```python
from build123d import *

# Parameters (mm, degrees)
MASS_DEPTH                = 6.35
SKETCH4_R                 = 9.271
CUT_EXTRUDE1_DEPTH        = 54.623672769
SKETCH3_W                 = 9.525
SKETCH3_H                 = 12.7
CUT_EXTRUDE2_DEPTH        = 54.623672769
LPATTERN1_COUNT           = 2
LPATTERN1_PITCH           = 19.05
CAVITY1_START             = -19.1516
CAVITY1_OUTLINE_W         = 11.1125
CAVITY1_OUTLINE_H         = 6.35
CAVITY1_DEPTH             = 6.35
CAVITY1_START_2           = 12.7
CAVITY1_2_OUTLINE_W       = 11.1125
CAVITY1_2_OUTLINE_H       = 6.35
CAVITY1_2_DEPTH           = 6.35
SKETCH5_R                 = 7.9375
CUT_EXTRUDE3_DEPTH        = 54.623672769
F_6_32_TAPPED_HOLE1_D     = 2.7051
F_6_32_TAPPED_HOLE1_DEPTH = 152.4
F_6_32_TAPPED_HOLE1_TIP   = 0.81269403


# Read off the part's stored shape, not the designer's step: Cavity1
with BuildPart() as part:
    # Sketch1 → Mass (new body)
    with BuildSketch(Plane.XY):
        with BuildLine():
            Line((-19.05, -23.8125), (19.05, -23.8125))
            Line((19.05, -23.8125), (19.05, 23.8125))
            Line((19.05, 23.8125), (-19.05, 23.8125))
            Line((-19.05, 23.8125), (-38.68314018, 14.281008096))
            ThreePointArc((-38.68314018, 14.281008096), (-47.625, 0), (-38.68314018, -14.281008096))
            Line((-38.68314018, -14.281008096), (-19.05, -23.8125))
        make_face()
    extrude(amount=MASS_DEPTH)

    # Sketch4 → Cut-Extrude1 (cut, through all)
    with BuildSketch(Plane(origin=(0, 0, 0), x_dir=(-1, 0, 0), z_dir=(0, 0, -1))):
        with Locations((31.75, 0)):
            Circle(SKETCH4_R)
    extrude(amount=-CUT_EXTRUDE1_DEPTH, mode=Mode.SUBTRACT)

    # Sketch3 → Cut-Extrude2 (cut, through all)
    with BuildSketch(Plane(origin=(0, 0, 0), x_dir=(-1, 0, 0), z_dir=(0, 0, -1))):
        with Locations((-14.2875, 23.8125)):
            Rectangle(SKETCH3_W, SKETCH3_H)
        with Locations((-14.2875, -23.8125)):
            Rectangle(SKETCH3_W, SKETCH3_H)
    cut_extrude2 = extrude(amount=-CUT_EXTRUDE2_DEPTH, mode=Mode.SUBTRACT)

    # LPattern1: Cut-Extrude2 ×2
    with Locations(*[(-i * LPATTERN1_PITCH, 0, 0) for i in range(1, LPATTERN1_COUNT)]):
        add(cut_extrude2, mode=Mode.SUBTRACT)

    # Cavity1 outline → Cavity1 (cut)
    with BuildSketch(Plane.YZ.offset(CAVITY1_START)):
        with Locations((-11.90625, 3.175)):
            Rectangle(CAVITY1_OUTLINE_W, CAVITY1_OUTLINE_H)
        with Locations((11.90625, 3.175)):
            Rectangle(CAVITY1_OUTLINE_W, CAVITY1_OUTLINE_H)
    extrude(amount=CAVITY1_DEPTH, mode=Mode.SUBTRACT)

    # Cavity1 2 outline → Cavity1 2 (cut)
    with BuildSketch(Plane.YZ.offset(CAVITY1_START_2)):
        with Locations((-11.90625, 3.175)):
            Rectangle(CAVITY1_2_OUTLINE_W, CAVITY1_2_OUTLINE_H)
        with Locations((11.90625, 3.175)):
            Rectangle(CAVITY1_2_OUTLINE_W, CAVITY1_2_OUTLINE_H)
    extrude(amount=CAVITY1_2_DEPTH, mode=Mode.SUBTRACT)

    # Sketch5 → Cut-Extrude3 (cut, through all)
    with BuildSketch(Plane(origin=(0, 0, 0), x_dir=(-1, 0, 0), z_dir=(0, 0, -1))):
        Circle(SKETCH5_R)
    extrude(amount=-CUT_EXTRUDE3_DEPTH, mode=Mode.SUBTRACT)

    # #6-32 Tapped Hole1
    with Locations(Plane(origin=(0, 0, 0), x_dir=(-1, 0, 0), z_dir=(0, 0, -1))):
        with Locations((23.059852363, -17.521321241), (12.169849394, 20.6375)):
            Hole(F_6_32_TAPPED_HOLE1_D / 2, depth=F_6_32_TAPPED_HOLE1_DEPTH)
            with Locations((0, 0, -(F_6_32_TAPPED_HOLE1_DEPTH + F_6_32_TAPPED_HOLE1_TIP / 2))):  # 118° drill point
                Cone(0, F_6_32_TAPPED_HOLE1_D / 2, F_6_32_TAPPED_HOLE1_TIP, mode=Mode.SUBTRACT)


solid = part.part
```
Model file for the job. Use its own axes, mm. A direction names the side the tool comes from. Give positions to 0.01 mm unless a question says otherwise; leave off trailing zeros. Write each loop counter-clockwise with the first axis right and the second up, starting at its lowest first coordinate (ties: lowest second). Pieces come first, ordered by that corner, then holes. Notation, with made-up numbers: (13, 86) -> (51, 86) arc R7 cw to (51, 99) -> close; hole circle Ø6 at (-0.5, 1). An arc over 180 degrees is marked (long way). Use CSV: the item, a comma, the result in double quotes. Start each with the question number.
1) Cut at A-A on y = 0. Count the separate pieces of the cut face and the enclosed holes in it, plus the area to 3 significant figures.
2) Two-plate mould, pull along X, no slides. Class faces 1 (the flat face through (-9.525, 21, 3)), 2 (the flat face through (12.7, 12, 3)), 3 (the flat face through (-16, 6.35, 3)), 4 (the flat face through (-29, -18.98, 3.13)): released by +X, released by -X, zero draft, split by the parting line, or undercut.
3) Cut at B-B on x = 2. List the corners of the cut face in (y, z).
4) Pin check, flat tips, straight feed: P1, Ø3, axis at y = -11.5, z = 2, coming from the +X side; P2, Ø4, axis at x = -4.5, y = -3.5, coming from the -Z side; P3, Ø1.9, axis at x = 16.5, z = 1.5, coming from the -Y side; P4, Ø3, axis at y = -21.5, z = 2.5, coming from the -X side. Stop position of each tip, or through.
5) Drill centre lines: L1, parallel to Y at x = -14, z = 4.5; L2, parallel to X at y = -7, z = 5.5; L3, parallel to X at y = 1, z = 2.5. Where is each one in solid material? Low to high.
6) Tool access for faces 5 (the flat face through (11, -17.462, 3)), 6 (the flat face through (11, 17.462, 3)), 7 (the flat face through (0, 21, 3)): list every direction of +Z, -Z, +X, -X, +Y, -Y with a clear straight run to the whole face (end or side of a thin tool).
7) Cut at C-C on y = -15. List the corners of the cut face in (x, z), plus the area to 3 significant figures.
Final values:
1,separate pieces,"3"
1,enclosed holes,"0"
1,area,"205 mm2"
2,face 1,"undercut"
2,face 2,"released by +X"
2,face 3,"undercut"
2,face 4,"released by -X"
3,outline,"(-23.81, 0) -> (-7.68, 0) -> (-7.68, 6.35) -> (-23.81, 6.35) -> close; (7.68, 0) -> (23.81, 0) -> (23.81, 6.35) -> (7.68, 6.35) -> close"
4,P1,"stops at x = 12.7"
4,P2,"passes through"
4,P3,"stops at y = -6.35"
4,P4,"stops at x = -26.9"
5,L1,"y = -23.81 to -17.46, -6.35 to 6.35, 17.46 to 23.81"
5,L2,"x = -46 to -37.83, -25.67 to -19.15, -12.8 to -3.74, 3.74 to 12.7"
5,L3,"x = -47.59 to -40.97, -22.53 to -7.87, 7.87 to 19.05"
6,face 5,"+Z, -Z, +X, -Y"
6,face 6,"+Z, -Z, +X, +Y"
6,face 7,"+Z, -Z, +Y"
7,outline,"(-37.2, 0) -> (-19.15, 0) -> (-19.15, 6.35) -> (-37.2, 6.35) -> close; (-12.8, 0) -> (12.7, 0) -> (12.7, 6.35) -> (-12.8, 6.35) -> close"
7,area,"277 mm2"
